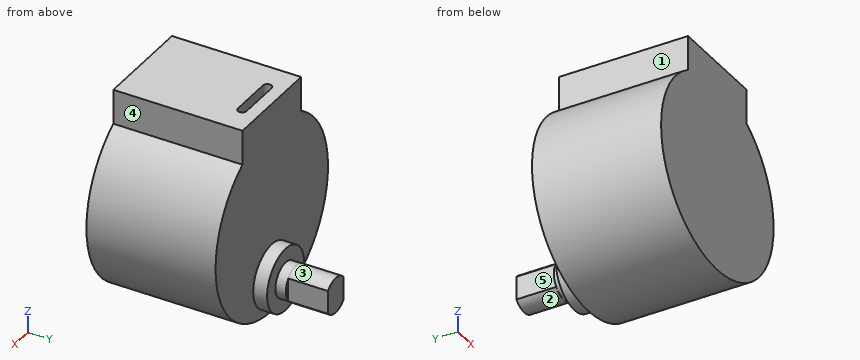
```python
from build123d import *

# Parameters (mm, degrees)
BOSS_EXTRUDE1_DEPTH = 18.8722
SKETCH3_R           = 4.5974
SKETCH3_R_2         = 2.54
BOSS_EXTRUDE2_DEPTH = 2.032
SKETCH3_2_R         = 4.5974
SKETCH3_2_R_2       = 2.54
BOSS_EXTRUDE3_DEPTH = 2.032
SKETCH4_R           = 2.54
BOSS_EXTRUDE4_DEPTH = 3.556
BOSS_EXTRUDE5_DEPTH = 5.8039
CUT_EXTRUDE1_DEPTH  = 7.62


with BuildPart() as part:
    # Sketch1 → Boss-Extrude1 (new body)
    with BuildSketch(Plane(origin=(0, 0, 0), x_dir=(1, 0, 0), z_dir=(0, 1, 0))):
        with BuildLine():
            Line((-7.28345, -11.921084519), (-7.28345, -17.001084519))
            Line((-7.28345, -17.001084519), (7.28345, -17.001084519))
            Line((7.28345, -17.001084519), (7.28345, -11.921084519))
            ThreePointArc((7.28345, -11.921084519), (0, 13.97), (-7.28345, -11.921084519))
        make_face()
    extrude(amount=BOSS_EXTRUDE1_DEPTH)

    # Sketch3 → Boss-Extrude2 (add)
    with BuildSketch(Plane(origin=(0, 18.8722, 0), x_dir=(1, 0, 0), z_dir=(0, 1, 0))):
        with Locations(Location((0.01905, 8.585233697, 0), (0, 0, 270))):
            Circle(SKETCH3_R)
        with Locations(Location((0.01905, 8.585233697, 0), (0, 0, 270))):
            Circle(SKETCH3_R_2, mode=Mode.SUBTRACT)
    extrude(amount=BOSS_EXTRUDE2_DEPTH)

    # Sketch3_2 → Boss-Extrude3 (add)
    with BuildSketch(Plane(origin=(0, 18.8722, 0), x_dir=(1, 0, 0), z_dir=(0, 1, 0))):
        with Locations(Location((0.01905, 8.585233697, 0), (0, 0, 270))):
            Circle(SKETCH3_2_R)
        with Locations(Location((0.01905, 8.585233697, 0), (0, 0, 270))):
            Circle(SKETCH3_2_R_2, mode=Mode.SUBTRACT)
    extrude(amount=BOSS_EXTRUDE3_DEPTH)

    # Sketch4 → Boss-Extrude4 (add)
    with BuildSketch(Plane(origin=(0, 18.8722, 0), x_dir=(1, 0, 0), z_dir=(0, 1, 0))):
        with Locations(Location((0.01905, 8.585233697, 0), (0, 0, 270))):
            Circle(SKETCH4_R)
    extrude(amount=BOSS_EXTRUDE4_DEPTH)

    # Sketch5 → Boss-Extrude5 (add)
    with BuildSketch(Plane(origin=(0, 22.4282, 0), x_dir=(1, 0, 0), z_dir=(0, 1, 0))):
        with BuildLine():
            Line((-1.921484266, 10.287033697), (-1.921484266, 6.883433697))
            ThreePointArc((-1.921484266, 6.883433697), (0.01905, 6.00418808), (1.959584266, 6.883433697))
            Line((1.959584266, 6.883433697), (1.959584266, 10.287033697))
            ThreePointArc((1.959584266, 10.287033697), (0.01905, 11.166279314), (-1.921484266, 10.287033697))
        make_face()
    extrude(amount=BOSS_EXTRUDE5_DEPTH)

    # Sketch6 → Cut-Extrude1 (cut)
    with BuildSketch(Plane.XY.offset(17.001084519)):
        with BuildLine():
            Line((-3.15595, 16.994300905), (3.06705, 16.994300905))
            ThreePointArc((3.06705, 16.994300905), (3.70205, 16.359300905), (3.06705, 15.724300905))
            Line((3.06705, 15.724300905), (-3.15595, 15.724300905))
            ThreePointArc((-3.15595, 15.724300905), (-3.79095, 16.359300905), (-3.15595, 16.994300905))
        make_face()
    extrude(amount=-CUT_EXTRUDE1_DEPTH, mode=Mode.SUBTRACT)


solid = part.part
```
Geometry check sheet. Reference: the model listing, model coordinates, mm. Face numbers are marked on the shaded views. A direction names the side the tool comes from. Coordinates: 2 decimals unless noted, no trailing zeros. Write each loop counter-clockwise with the first axis right and the second up, starting at its lowest first coordinate (ties: lowest second). Pieces come first, ordered by that corner, then holes. Notation, with made-up numbers: M -3.5,30 L 23.5,30 A31 ccw 23.5,54 Z; hole C 51.5,25.25 d10. An arc over 180 degrees is marked long. One line per item, written item: value. Start each with the question number.
(1) Sectioned sample at C-C, the plane y = 3.25. Enter the section's corners in (x, z).
(2) Scan lines: line 1 along Y through (x, z) = (7, 3); line 2 along Y through (x, z) = (3, 12); line 3 along X through (y, z) = (16.75, 14). Record each from-to range of solid material in increasing order. Write a range as [from, to].
(3) Depth check by flat-ended pin: pin 1 (8.5 mm diameter, centred on x = -1.5, z = 5.5, fed in from +Y); pin 2 (1 mm diameter, centred on x = 3.5, z = 5.5, fed in from -Y); pin 3 (1 mm diameter, centred on y = 25.5, z = -9, fed in from +X); pin 4 (4 mm diameter, centred on y = 7, z = 15.5, fed in from +X). Enter the tip coordinate at first touch or a pass-through.
(4) Tool access check on the marked faces 1, 2, 3, 4 and 5. Record the directions out of +Z, -Z, +X, -X, +Y, -Y that give a thin tool (end or side, any length) a straight path to the whole face; none if there is none.
(5) Sectioned sample at D-D, the plane y = 20. Enter the section's corners in (x, z), and give its area (3 significant figures).
(6) Sectioned sample at B-B, the plane z = 0. Enter the section's corners in (x, y), and give its area (3 significant figures).
(7) Sectioned sample at A-A, the plane z = 14. Enter the section's corners in (x, y) (3 decimals), and give its area (3 significant figures).
Filled sheet:
1. outline: M -7.28,11.92 A13.97 ccw long 7.28,11.92 L 7.28,17 L -7.28,17 Z
2. line 1: [0, 18.87]
2. line 2: [0, 15.72], [16.99, 18.87]
2. line 3: [-7.28, -3.66], [3.57, 7.28]
3. pin 1: y = 18.87
3. pin 2: y = 0
3. pin 3: x = 1.96
3. pin 4: x = 7.28
4. face 1: +Z, -X, +Y, -Y
4. face 2: -Z, +Y
4. face 3: +Z, +Y
4. face 4: +Z, +X, +Y, -Y
4. face 5: +Z, -Z, -X, +Y
5. outline: C 0.02,-8.59 d9.19
5. area: 66.4 mm²
6. outline: M -13.97,0 L 13.97,0 L 13.97,18.87 L -13.97,18.87 Z
6. area: 527 mm²
7. outline: M -7.283,0 L 7.283,0 L 7.283,18.872 L -7.283,18.872 Z; hole M -3.156,15.724 L 3.067,15.724 A0.635 ccw 3.067,16.994 L -3.156,16.994 A0.635 ccw Z
7. area: 266 mm²
